The listing builds one solid part. Answer for the finished solid, in the listing's coordinates (mm). Round coordinates to 2 decimals unless told otherwise and drop trailing zeros. Write each loop counter-clockwise with the first axis right and the second up, starting at its lowest first coordinate (ties: lowest second). Pieces come first, ordered by that corner, then holes. Notation, with made-up numbers: (-1.5, 87) - (22.5, 87) arc R26 ccw to (22.5, 123) - close; hole circle Ø9 at (71, 1). An arc over 180 degrees is marked (long way). Use a Markdown table: item, result. Add a question column.
1) A cutting plane is placed at A-A (x = -114). Give the vertices of the cut face in (y, z).
2) Find the intervals of material crossed by probe 1 along Z at (x, y) = (-140, -4); probe 2 along Z at (x, y) = (-140, -6.5); probe 3 along Y at (x, z) = (-64.5, 1.5), in increasing order. Write a range as from..to.
3) This flat-tipped pin is pushed along its axis until it touches: P1, Ø2.5, axis at x = 60, z = 5, coming from the -Y side. Where does it stop, or does it pass through?
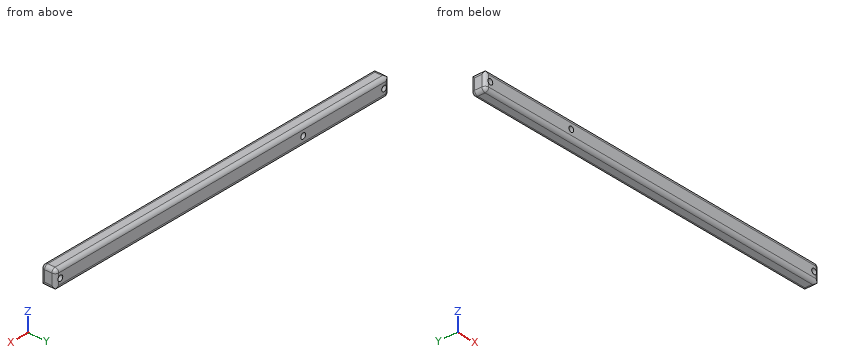
```python
from build123d import *

# Parameters (mm, degrees)
F0_W         = 206
F0_H         = 10
F0_R         = 1.5
F1_DEPTH     = 8
F2_T1_DEPTH  = 4
F2_T3_DEPTH  = 18
F2_T5_DEPTH  = 209
F2_T7_DEPTH  = 13
F2_S11_W     = 2
F2_S11_H     = 2
F2_T12_DEPTH = 2
F2_S17_W     = 2
F2_S17_H     = 2
F2_T18_DEPTH = 2
F3_T1_DEPTH  = 11
F3_T3_DEPTH  = 4
F3_T5_DEPTH  = 207
F3_S9_W      = 2.04
F3_S9_H      = 2.04
F3_T10_DEPTH = 2.04
F3_S15_W     = 2.04
F3_S15_H     = 2.04
F3_T16_DEPTH = 2.04


# Not quite as in the source:
# - a fillet or chamfer that OpenCascade refuses, or shapes differently, is made with other operations: its cross-section is extruded or revolved along the edge and cut away or added


with BuildPart() as f1:
    # F0 (on Front) → F1 (new body)
    with BuildSketch(Plane.XZ):
        with Locations((-40, 5)):
            Rectangle(F0_W, F0_H)
        with Locations((-140, 5)):
            Circle(F0_R, mode=Mode.SUBTRACT)
        with Locations((-90, 5)):
            Circle(F0_R, mode=Mode.SUBTRACT)
        with Locations((60, 5)):
            Circle(F0_R, mode=Mode.SUBTRACT)
    extrude(amount=F1_DEPTH)

    # F2: fillet of radius 2 on 7 edges, made by hand

    # F2_s2 → F2_t1 (cut)
    with BuildSketch(Plane.XZ.offset(2)):
        with BuildLine():
            ThreePointArc((63, 8), (62.4142135624, 9.4142135624), (61, 10))
            Line((61, 10), (63, 10))
            Line((63, 10), (63, 8))
        make_face()
    extrude(amount=F2_T1_DEPTH, mode=Mode.SUBTRACT)

    # F2_s4 → F2_t3 (cut)
    with BuildSketch(Plane.XZ.offset(-5)):
        with BuildLine():
            ThreePointArc((-143, 8), (-142.4142135624, 9.4142135624), (-141, 10))
            Line((-141, 10), (-143, 10))
            Line((-143, 10), (-143, 8))
        make_face()
        with BuildLine():
            ThreePointArc((61, 0), (62.4142135624, 0.5857864376), (63, 2))
            Line((63, 2), (63, 0))
            Line((63, 0), (61, 0))
        make_face()
    extrude(amount=F2_T3_DEPTH, mode=Mode.SUBTRACT)

    # F2_s6 → F2_t5 (cut)
    with BuildSketch(Plane.YZ.offset(-148)):
        with BuildLine():
            ThreePointArc((-2, 10), (-0.5857864376, 9.4142135624), (0, 8))
            Line((0, 8), (0, 10))
            Line((0, 10), (-2, 10))
        make_face()
        with BuildLine():
            ThreePointArc((-6, 10), (-7.4142135624, 9.4142135624), (-8, 8))
            Line((-8, 8), (-8, 10))
            Line((-8, 10), (-6, 10))
        make_face()
    extrude(amount=F2_T5_DEPTH, mode=Mode.SUBTRACT)

    # F2_s8 → F2_t7 (cut)
    with BuildSketch(Plane.XY.offset(-5)):
        with BuildLine():
            ThreePointArc((63, -2), (62.4142135624, -0.5857864376), (61, 0))
            Line((61, 0), (63, 0))
            Line((63, 0), (63, -2))
        make_face()
        with BuildLine():
            ThreePointArc((63, -6), (62.4142135624, -7.4142135624), (61, -8))
            Line((61, -8), (63, -8))
            Line((63, -8), (63, -6))
        make_face()
    extrude(amount=F2_T7_DEPTH, mode=Mode.SUBTRACT)


with BuildPart() as f2_tool10:
    # F2_s11 → F2_t12 (new body)
    with BuildSketch(Plane.YZ.offset(61)):
        with Locations((-1, 9)):
            Rectangle(F2_S11_W, F2_S11_H)
    extrude(amount=F2_T12_DEPTH)

    # F2_s13 → F2_t14 (revolve, cut)
    with BuildSketch(Plane(origin=(61, -2, 8), x_dir=(0, -0.7071067812, -0.7071067812), z_dir=(0, -0.7071067812, 0.7071067812))):
        with BuildLine():
            ThreePointArc((0, -2), (2, 0), (0, 2))
            Line((0, 2), (0, -2))
        make_face()
    revolve(axis=Axis((61, -2, 8), (1, 0, 0)), mode=Mode.SUBTRACT)


with BuildPart() as f1_1:
    add(f1.part)

    # F2_t9: cut F2_tool10
    add(f2_tool10.part, mode=Mode.SUBTRACT)


with BuildPart() as f2_tool16:
    # F2_s17 → F2_t18 (new body)
    with BuildSketch(Plane.XZ.offset(6)):
        with Locations((62, 9)):
            Rectangle(F2_S17_W, F2_S17_H)
    extrude(amount=F2_T18_DEPTH)

    # F2_s19 → F2_t20 (revolve, cut)
    with BuildSketch(Plane(origin=(61, -6, 8), x_dir=(-0.7071067812, 0, -0.7071067812), z_dir=(-0.7071067812, 0, 0.7071067812))):
        with BuildLine():
            ThreePointArc((0, -2), (2, 0), (0, 2))
            Line((0, 2), (0, -2))
        make_face()
    revolve(axis=Axis((61, -6, 8), (0, -1, 0)), mode=Mode.SUBTRACT)


with BuildPart() as f1_2:
    add(f1_1.part)

    # F2_t15: cut F2_tool16
    add(f2_tool16.part, mode=Mode.SUBTRACT)

    # F3: fillet of radius 2 on 7 edges, made by hand

    # F3_s2 → F3_t1 (cut)
    with BuildSketch(Plane.XY.offset(2)):
        with BuildLine():
            ThreePointArc((-143, -2), (-142.4142135624, -0.5857864376), (-141, 0))
            Line((-141, 0), (-143, 0))
            Line((-143, 0), (-143, -2))
        make_face()
        with BuildLine():
            ThreePointArc((-143, -6), (-142.4142135624, -7.4142135624), (-141, -8))
            Line((-141, -8), (-143, -8))
            Line((-143, -8), (-143, -6))
        make_face()
    extrude(amount=F3_T1_DEPTH, mode=Mode.SUBTRACT)

    # F3_s4 → F3_t3 (cut)
    with BuildSketch(Plane.XZ.offset(2)):
        with BuildLine():
            ThreePointArc((-143, 2), (-142.4142135624, 0.5857864376), (-141, 0))
            Line((-141, 0), (-143, 0))
            Line((-143, 0), (-143, 2))
        make_face()
    extrude(amount=F3_T3_DEPTH, mode=Mode.SUBTRACT)

    # F3_s6 → F3_t5 (cut)
    with BuildSketch(Plane.YZ.offset(-141)):
        with BuildLine():
            ThreePointArc((0, 2), (-0.5857864376, 0.5857864376), (-2, 0))
            Line((-2, 0), (0, 0))
            Line((0, 0), (0, 2))
        make_face()
        with BuildLine():
            ThreePointArc((-6, 0), (-7.4142135624, 0.5857864376), (-8, 2))
            Line((-8, 2), (-8, 0))
            Line((-8, 0), (-6, 0))
        make_face()
    extrude(amount=F3_T5_DEPTH, mode=Mode.SUBTRACT)


with BuildPart() as f3_tool8:
    # F3_s9 → F3_t10 (new body)
    with BuildSketch(Plane.YZ.offset(-141)):
        with Locations((-0.98, 0.98)):
            Rectangle(F3_S9_W, F3_S9_H)
    extrude(amount=-F3_T10_DEPTH)

    # F3_s11 → F3_t12 (revolve, cut)
    with BuildSketch(Plane(origin=(-141, -2, 2), x_dir=(0, -0.7071067812, 0.7071067812), z_dir=(0, -0.7071067812, -0.7071067812))):
        with BuildLine():
            ThreePointArc((0, -2), (2, 0), (0, 2))
            Line((0, 2), (0, -2))
        make_face()
    revolve(axis=Axis((-141, -2, 2), (-1, 0, 0)), mode=Mode.SUBTRACT)


with BuildPart() as f1_3:
    add(f1_2.part)

    # F3_t7: cut F3_tool8
    add(f3_tool8.part, mode=Mode.SUBTRACT)


with BuildPart() as f3_tool14:
    # F3_s15 → F3_t16 (new body)
    with BuildSketch(Plane.YZ.offset(-141)):
        with Locations((-7.02, 0.98)):
            Rectangle(F3_S15_W, F3_S15_H)
    extrude(amount=-F3_T16_DEPTH)

    # F3_s17 → F3_t18 (revolve, cut)
    with BuildSketch(Plane(origin=(-141, -6, 2), x_dir=(0, 0.7071067812, 0.7071067812), z_dir=(0, -0.7071067812, 0.7071067812))):
        with BuildLine():
            ThreePointArc((0, -2), (2, 0), (0, 2))
            Line((0, 2), (0, -2))
        make_face()
    revolve(axis=Axis((-141, -6, 2), (-1, 0, 0)), mode=Mode.SUBTRACT)


with BuildPart() as f1_4:
    add(f1_3.part)

    # F3_t13: cut F3_tool14
    add(f3_tool14.part, mode=Mode.SUBTRACT)


solid = f1_4.part
```
Entries:
| question | item | result |
|---|---|---|
| 1 | outline | (-8, 2) arc R2 ccw to (-6, 0) - (-2, 0) arc R2 ccw to (0, 2) - (0, 8) arc R2 ccw to (-2, 10) - (-6, 10) arc R2 ccw to (-8, 8) - close |
| 2 | probe 1 | z = 0..3.5, 6.5..10 |
| 2 | probe 2 | z = 0.06..3.5, 6.5..9.94 |
| 2 | probe 3 | y = -7.94..-0.06 |
| 3 | P1 | passes through |
